Geometry: final body of the model. Coordinates: model frame, mm. Face numbers are marked on the shaded views. Round coordinates to 2 decimals unless told otherwise and drop trailing zeros. Write each loop counter-clockwise with the first axis right and the second up, starting at its lowest first coordinate (ties: lowest second). Pieces come first, ordered by that corner, then holes. Notation, with made-up numbers: (53.5, -21.5) - (76.5, -21.5) arc R22 ccw to (76.5, 4.5) - close; hole circle Ø3 at (-2.5, -14.5). An arc over 180 degrees is marked (long way). Write each question's results on one line, items separated by ' | '.
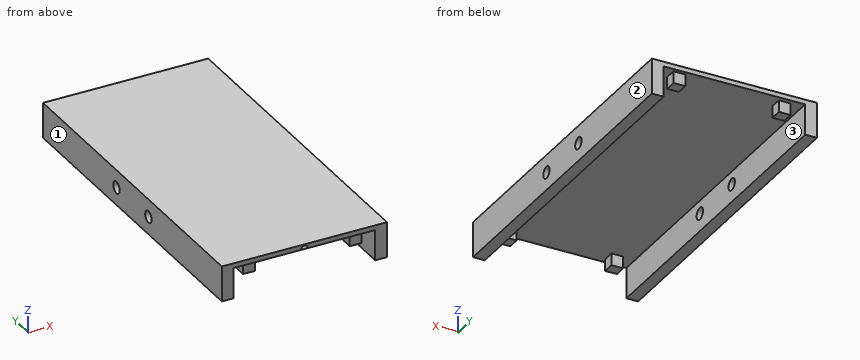
from build123d import *

# Parameters (mm, degrees)
SKETCH2_W           = 70
SKETCH2_H           = 140
BOSS_EXTRUDE1_DEPTH = 15
SKETCH3_W           = 60
SKETCH3_H           = 130
CUT_EXTRUDE1_DEPTH  = 12.5
SKETCH4_W           = 60
SKETCH4_H           = 13
CUT_EXTRUDE2_DEPTH  = 141
SKETCH7_R           = 2.5
CUT_EXTRUDE5_DEPTH  = 71
CUT_REVOLVE1_ANGLE  = 30
SKETCH36_W          = 5
SKETCH36_H          = 5
BOSS_EXTRUDE2_DEPTH = 5


with BuildPart() as part:
    # Sketch2 → Boss-Extrude1 (new body)
    with BuildSketch(Plane.XY):
        with Locations((35, 368.888888889)):
            Rectangle(SKETCH2_W, SKETCH2_H)
    extrude(amount=-BOSS_EXTRUDE1_DEPTH)

    # Sketch3 → Cut-Extrude1 (cut)
    with BuildSketch(Plane(origin=(0, 0, -15), x_dir=(-1, 0, 0), z_dir=(0, 0, -1))):
        with Locations((-35, 368.888888889)):
            Rectangle(SKETCH3_W, SKETCH3_H)
    extrude(amount=-CUT_EXTRUDE1_DEPTH, mode=Mode.SUBTRACT)

    # Sketch4 → Cut-Extrude2 (cut, through all)
    with BuildSketch(Plane(origin=(0, 438.888888889, 0), x_dir=(1, 0, 0), z_dir=(0, 1, 0))):
        with Locations((35, 8.5)):
            Rectangle(SKETCH4_W, SKETCH4_H)
    extrude(amount=-CUT_EXTRUDE2_DEPTH, mode=Mode.SUBTRACT)

    # Sketch7 → Cut-Extrude5 (cut, through all)
    with BuildSketch(Plane.ZY):
        with Locations((-7.5, 381.388888889)):
            Circle(SKETCH7_R)
        with Locations((-7.5, 356.388888889)):
            Circle(SKETCH7_R)
    extrude(amount=-CUT_EXTRUDE5_DEPTH, mode=Mode.SUBTRACT)

    # Sketch32 → Cut-Revolve1 (revolve, cut)
    with BuildSketch(Plane.XZ.offset(-298.888888889)):
        with BuildLine():
            Line((33.5, -2), (36.5, -2))
            ThreePointArc((36.5, -2), (35, -0.5), (33.5, -2))
        make_face()
    revolve(axis=Axis((33.5, 298.888888889, -2), (-1, 0, 0)), revolution_arc=CUT_REVOLVE1_ANGLE, mode=Mode.SUBTRACT)

    # Sketch36 → Boss-Extrude2 (add)
    with BuildSketch(Plane(origin=(0, 0, -2), x_dir=(-1, 0, 0), z_dir=(0, 0, -1))):
        with Locations((-57.5, 434.888888889)):
            Rectangle(SKETCH36_W, SKETCH36_H)
        Polygon((-10.145008864, 431.85472827), (-15.143861036, 431.961858829), (-15.036730477, 436.960711001), (-10.037878305, 436.853580442), align=None)
        Polygon((-10.145008864, 305.923049508), (-15.143861036, 305.815918949), (-15.036730477, 300.817066777), (-10.037878305, 300.924197336), align=None)
        with Locations((-57.5, 302.888888889)):
            Rectangle(SKETCH36_W, SKETCH36_H)
    extrude(amount=BOSS_EXTRUDE2_DEPTH)


solid = part.part
Q1. Mould query, pull axis X, two halves, no side actions, for the marked faces 1, 2 and 3. Classes: pulls with the +X half, pulls with the -X half, needs draft (parallel to the pull), parting line crosses it, or undercut.
Answer block:
face 1: pulls with the -X half | face 2: pulls with the +X half | face 3: undercut
Q2. Section query A-A, the plane x = 58. Return loops of the section in (y, z).
Answer block:
outline: (298.89, -2) - (300.39, -2) - (300.39, -7) - (305.39, -7) - (305.39, -2) - (432.39, -2) - (432.39, -7) - (437.39, -7) - (437.39, -2) - (438.89, -2) - (438.89, 0) - (298.89, 0) - close
Q3. Ray query, line 1 along Y through (x, z) = (66.1, -7.5); line 2 along X through (y, z) = (433, -3.5); line 3 along X through (y, z) = (372.5, -11.5). Return the intervals inside material, ascending.
Answer block:
line 1: 298.89 to 353.89, 358.89 to 378.89, 383.89 to 438.89 | line 2: 0 to 5, 10.12 to 15.12, 55 to 60, 65 to 70 | line 3: 0 to 5, 65 to 70
Q4. Pin query (flat end, axial travel): pin 1 (5.5 mm diameter, centred on x = 58, z = -5, fed in from -Y); pin 2 (2.5 mm diameter, centred on x = 11.5, y = 303, fed in from -Z). Return the tip coordinate at first contact, or that it passes through.
Answer block:
pin 1: y = 300.39 | pin 2: z = -7
Q5. Section query B-B, the plane y = 350.5. Return loops of the section in (x, z), plus the area to 3 significant figures.
Answer block:
outline: (0, -15) - (5, -15) - (5, -2) - (65, -2) - (65, -15) - (70, -15) - (70, 0) - (0, 0) - close | area: 270 mm2
Q6. Section query C-C, the plane x = 38.5. Return loops of the section in (y, z).
Answer block:
outline: (298.89, -2) - (438.89, -2) - (438.89, 0) - (298.89, 0) - close
